Autodesk Inventor part; units mm, degrees
ref_plane "YZ Plane" through (0, 0, 0) normal (1, 0, 0) x (0, 1, 0)
ref_plane "XZ Plane" through (0, 0, 0) normal (0, 1, 0) x (-1, 0, 0)
ref_plane "XY Plane" through (0, 0, 0) normal (0, 0, 1) x (1, 0, 0)
sketch "Sketch1" plane through (0, 0, 0) normal (0, 1, 0) x (-1, 0, 0)
  line L0 (16.2222, 35.2121) -> (-14.7778, 35.2121)
  line L1 (-14.7778, 35.2121) -> (-14.7778, -34.7879)
  line L2 (-14.7778, -34.7879) -> (16.2222, -34.7879)
  line L3 (16.2222, -34.7879) -> (16.2222, 35.2121)
  point P0 (0, 0)
  dimension "d0" = 70
  dimension "d1" = 31
extrude "Extrusion1" add sketch "Sketch1" along normal blind 60
sketch "Sketch2" plane through (0, 60, 0) normal (0, 1, 0) x (1, 0, 0)
  line L0 (0, -17.35) -> (0, 17.35)
  point P0 (0, 0)
  point P1 (0, 0)
  dimension "d4" = 34.7
sketch "Sketch3" plane through (14.7778, 0, 35.2121) normal (1, 0, 0) x (0, 0, -1)
  circle A0 centre (35.2121, 37.6844) radius 27.5
  point P0 (35.2121, 0)
  dimension "d5" = 55
hole "Hole1" at (14.7778, 37.6844, 0) direction (-1, 0, 0) diameter 55 end through all
sketch "Sketch4" plane through (0, 60, 0) normal (0, 1, 0) x (1, 0, 0)
  line L0 (14.7778, -16.0705) -> (-16.2222, -16.0705)
  circle A0 centre (0, -16.0705) radius 4
  point P0 (0, 0)
  dimension "d13" = 8
sketch "Sketch5" plane through (0, 60, 0) normal (0, 1, 0) x (1, 0, 0)
  line L0 (-16.2222, 16.0705) -> (14.7778, 16.0705)
  circle A0 centre (0, 16.0705) radius 4
  point P0 (0, 0)
  dimension "d14" = 8
hole "Hole2" at (0, 60, 16.0705) direction (0, -1, 0) diameter 8 depth 8 tip angle 118
hole "Hole3" at (0, 60, -16.0705) direction (0, -1, 0) diameter 8 depth 8 tip angle 118
sketch "Sketch6" plane through (0, 60, 0) normal (0, 1, 0) x (1, 0, 0)
  arc A0 (-4, -16.0705) -> (4, -16.0705) centre (0, -16.0705) ccw
  line L0 (0, -20.0705) -> (14.7778, -20.0705)
  line L1 (14.7778, -20.0705) -> (14.7778, -16.0705)
  line L2 (14.7778, -16.0705) -> (0, -16.0705)
  line L3 (14.7778, -16.0705) -> (4, -16.0705)
  line L4 (0, -16.0705) -> (0, -20.0705)
  point P0 (0, 0)
extrude "Extrusion2" cut sketch "Sketch6" against normal blind 10 contours A0 L2 L1 L0
sketch "Sketch7" plane through (0, 60, 0) normal (0, 1, 0) x (1, 0, 0)
  arc A0 (4, 16.0705) -> (-4, 16.0705) centre (0, 16.0705) ccw
  line L0 (0, 20.0705) -> (14.7778, 20.0705)
  line L1 (14.7778, 16.0705) -> (14.7778, 34.7879)
  line L2 (14.7778, 20.0705) -> (14.7778, 16.0705)
  line L3 (14.7778, 16.0705) -> (0, 16.0705)
  line L4 (0, 16.0705) -> (0, 20.0705)
  point P0 (0, 0)
extrude "Extrusion3" cut sketch "Sketch7" against normal blind 10
properties part number "Noke_holder"
Geometry: final body of the model. Coordinates: model frame, mm. A direction names the side the tool comes from. Coordinates: 2 decimals unless noted, no trailing zeros. Loops run counter-clockwise (first coordinate to the right, second up) from the corner with the lowest first, then second, coordinate; pieces in that order, holes last. Notation, with made-up numbers: M -33,-6.75 L -4,-6.75 A19 cw -4,-2.75 Z; hole C 70.5,13.25 d11. An arc over 180 degrees is marked long. Put each result on its own line as item: value.
(1) Access query for faces 5 (the face through (14.778, 10, 1)), 6 (the face through (7, 58, -20.07)). Directions: +Z, -Z, +X, -X, +Y, -Y. A direction counts if a zero-diameter tool reaches every point of the face in a straight line with its end or side. Return the directions, or none.
Answer sheet:
face 5: +Z, -Z, +X, +Y, -Y
face 6: +X, +Y
(2) Cut plane D-D on z = 0. Return the cut outline in (x, y), then the cut area to 3 significant figures.
Answer sheet:
outline: M -16.22,0 L 14.78,0 L 14.78,10.18 L -16.22,10.18 Z
area: 316 mm^2
(3) Cut plane C-C on x = -8.5. Return the cut outline in (y, z), then the cut area to 3 significant figures.
Answer sheet:
outline: M 0,-34.79 L 60,-34.79 L 60,-16.07 A27.5 cw long 60,16.07 L 60,35.21 L 0,35.21 Z
area: 1,940 mm^2
(4) First-contact query: pin 1 (2 mm diameter, centred on x = -5.5, z = -10, fed in from +Y); pin 2 (8 mm diameter, centred on x = 3.5, z = -11, fed in from +Y); pin 3 (1.5 mm diameter, centred on x = -6, z = 9.5, fed in from +Y). Flat tips, straight axial feed; report the tip coordinate or a pass-through.
Answer sheet:
pin 1: stops at y = 12.48
pin 2: stops at y = 14.64
pin 3: stops at y = 12.17
(5) Material intervals for probe 1 along Z at (x, y) = (7, 37); probe 2 along Z at (x, y) = (9.5, 55.5); probe 3 along Y at (x, z) = (4, 0.5), sorted ascending.
Answer sheet:
probe 1: z = -34.79 to -27.49, 27.49 to 35.21
probe 2: z = -34.79 to -20.95, 20.95 to 35.21
probe 3: y = 0 to 10.19
(6) Cut plane B-B on z = -21. Return the cut outline in (x, y).
Answer sheet:
outline: M -16.22,0 L 14.78,0 L 14.78,19.93 L -16.22,19.93 Z; M -16.22,55.44 L 14.78,55.44 L 14.78,60 L -16.22,60 Z
(7) Cut plane A-A on y = 42. Return the cut outline in (x, z).
Answer sheet:
outline: M -16.22,-34.79 L 14.78,-34.79 L 14.78,-27.16 L -16.22,-27.16 Z; M -16.22,27.16 L 14.78,27.16 L 14.78,35.21 L -16.22,35.21 Z
(8) Draft query along Y for faces 1 (the face through (-1, 0, 1)), 2 (the face through (-0.94, 10.2, -0.97)), 3 (the face through (-16.222, 10, 0)), 4 (the face through (-1, 60, -25)). Return one class per face: pulls with the +Y half, pulls with the -Y half, needs draft (parallel to the pull), parting line crosses it, or undercut.
Answer sheet:
face 1: pulls with the -Y half
face 2: undercut
face 3: needs draft
face 4: pulls with the +Y half
